CAD build for the part. Positions are in the model's coordinates, mm. A direction names the side the tool comes from. Round coordinates to 2 decimals unless told otherwise and drop trailing zeros. Order: outer loops, then holes, each group sorted by start corner. A loop starts at its lowest first (then second) coordinate and runs counter-clockwise, first axis right, second up. Notation, with made-up numbers: M 7,-18 L 36,-18 A22 cw 36,17 Z; hole C -22,56 d6. An arc over 180 degrees is marked long. Answer as a JSON object with one key per item and string values.
Autodesk Inventor part; units mm, degrees
ref_plane "Work Plane1" through (8, 0, 0) normal (0, 0, -1) x (1, 0, 0)
ref_plane "YZ Plane" through (0, 0, 0) normal (1, 0, 0) x (0, 1, 0)
ref_plane "XZ Plane" through (0, 0, 0) normal (0, 1, 0) x (-1, 0, 0)
sketch "Sketch1" plane through (0, 0, 0) normal (0, 0, 1) x (1, 0, 0)
  line L0 (0, 0) -> (13, 0)
  line L1 (13, 0) -> (13, 3)
  line L2 (13, 3) -> (5, 3)
  line L3 (5, 3) -> (5, 4)
  line L4 (5, 4) -> (0, 4)
  line L5 (0, 4) -> (0, 0)
  line L6 (-2.6, 0) -> (15.6, 0)
  line L7 (0, -0.8) -> (0, 4.8)
  arc A0 (5, 3) -> (6, 3) centre (5.5, 3.866) ccw
  dimension "d0" = 5
  dimension "d1" = 8
  dimension "d2" = 6
  dimension "d3" = 8
  dimension "d14" = 1
  dimension "d15" = 1
revolve "Body" add sketch "Sketch1" angle 360 about axis through (0, 0, 0) along (1, 0, 0)
sketch "Sketch2" plane through (0, 0, 0) normal (-1, 0, 0) x (0, 0, 1)
  circle A0 centre (0, 0) radius 4
  line L0 (0, -5.6) -> (0, 5.6)
  line L1 (-5.6, 0) -> (5.6, 0)
  line L2 (-4, 0.5) -> (4, 0.5)
  line L3 (4, 0.5) -> (4, -0.5)
  line L4 (4, -0.5) -> (-4, -0.5)
  line L5 (-4, -0.5) -> (-4, 0.5)
  line L6 (-4, 0) -> (4, 0) construction
  line L7 (0, 0.5) -> (0, -0.5) construction
  dimension "d5" = 1
extrude "Slot" cut sketch "Sketch2" against normal blind 2 contours L1 L0 L2 A0 | L3 L4 A0 | A0 L4 L0 L1 | A0 L2 L3 | L1 A0 L2 L0 | L0 L4 A0 L1 | L5 L2 A0 | A0 L4 L5
chamfer "Chamfer1" distance 1 angle 45 3 edges at (0, 3, -2.6458) (0, 3, 2.6458) (0, -4, 0) measured on face at (3.3333, -1.7193, 3.6117)
thread "Thread"
chamfer "Chamfer2" distance 0.6135 distance2 0.6135 1 edges at (13, -3, 0) measured on face at (13, 0.7776, -0.4238)
revolve "Groove1" cut sketch "Sketch1" angle 360 about axis through (0, 0, 0) along (1, 0, 0) contours A0 L2
ref_plane "Work Plane1" through (8, 0, 0) normal (0, 0, -1) x (1, 0, 0)
equation "\"d0\" = KOH"
equation "\"d1\" = GEL"
equation "\"d2\" = NND"
equation "\"d3\" = KOD"
equation "\"d14\" = SBR"
equation "\"d15\" = SBR"
equation "\"d5\" = SBR"
equation "\"d6\" = STI"
equation "\"d8\" = PHH"
equation "\"d19\" = PHH"
equation "\"d10\" = GEL"
equation "\"d12\" = -0.5 * GD1 + 0.5 * NND"
equation "\"d13\" = GUL"
equation "\"NND\" = 6"
equation "\"GEL\" = 8"
equation "\"KOD\" = 8"
equation "\"KOH\" = 5"
equation "\"SBR\" = 1"
equation "\"GUL\" = 0.61345 * PTC"
equation "\"PHH\" = 1"
equation "\"GD1\" = THREADDIA - 1.2269 * PTC"
equation "\"STI\" = 2"
equation "\"THREADDIA\" = 6"
equation "\"TOA\" = 30deg"
equation "\"NLG\" = GEL"
equation "\"PTC\" = 1"
equation "\"GAL\" = 0.61345 * PTC"
properties part number "DIN 927 - M6 x 5-14H" material "Steel, Mild"
Item 1: Saw through at A-A on y = 0. List the corners of the cut face in (x, z).
Worked answers:
{"outline": "M 2,-4 L 5,-4 L 5,-3 A1 cw 6,-3 L 12.39,-3 L 13,-2.39 L 13,2.39 L 12.39,3 L 6,3 A1 cw 5,3 L 5,4 L 2,4 Z"}
Item 2: Saw through at D-D on x = 11. List the corners of the cut face in (y, z), and give its area (3 significant figures).
Worked answers:
{"outline": "C 0,0 d6", "area": "28.3 mm2"}
Item 3: Saw through at B-B on z = 0. List the corners of the cut face in (x, y), and give its area (3 significant figures).
Worked answers:
{"outline": "M 0,-3 L 1,-4 L 5,-4 L 5,-3 A1 cw 6,-3 L 12.39,-3 L 13,-2.39 L 13,2.39 L 12.39,3 L 6,3 A1 cw 5,3 L 5,4 L 1,4 L 0,3 L 0,0.5 L 2,0.5 L 2,-0.5 L 0,-0.5 Z", "area": "84.4 mm2"}
Item 4: 3-axis set-ups, long thin cutter, end or side, ignore diameter. For faces 1 (the flat face through (2, 0, 0)), 2 (the cylindrical face through (2.972, -0.867, 3.905)): which of +Z, -Z, +X, -X, +Y, -Y reach the whole face in a straight line?
Worked answers:
{"face 1": "+Z, -Z, -X", "face 2": "+X, -X"}
Item 5: Two-plate mould, pull along Y, no slides. Class faces 3 (the cylindrical face through (9, -3, 0)), 4 (the flat face through (5, 1, 3)), 5 (the flat face through (1, -0.5, 0)): released by +Y, released by -Y, zero draft, split by the parting line, or undercut.
Worked answers:
{"face 3": "split by the parting line", "face 4": "zero draft", "face 5": "undercut"}
Item 6: Saw through at C-C on x = 2.5. List the corners of the cut face in (y, z), and give its area (3 significant figures).
Worked answers:
{"outline": "C 0,0 d8", "area": "50.3 mm2"}
Item 7: Drop flat-ended pins along their axis: pin 1 Ø3 at (x, y) = (8.5, -3) entering from -Z; pin 2 Ø1.6 at (x, z) = (1.5, -1.5) entering from -Y; pin 3 Ø0.5 at (y, z) = (0, -1.5) entering from -X. Give the stop position or say it passes through.
Worked answers:
{"pin 1": "stops at z = -2.6", "pin 2": "stops at y = -3.94", "pin 3": "stops at x = 2"}
Item 8: Wall check: line 1 along Z through (x, y) = (8, 0.5); line 2 along Y through (x, z) = (1.25, 2.5); line 3 along Z through (x, y) = (2.25, 0.5). Give the ranges that are in metal, low to high. Write a range as [from, to].
Worked answers:
{"line 1": "z = [-2.96, 2.96]", "line 2": "y = [-3.12, -0.5], [0.5, 3.12]", "line 3": "z = [-3.97, 3.97]"}
